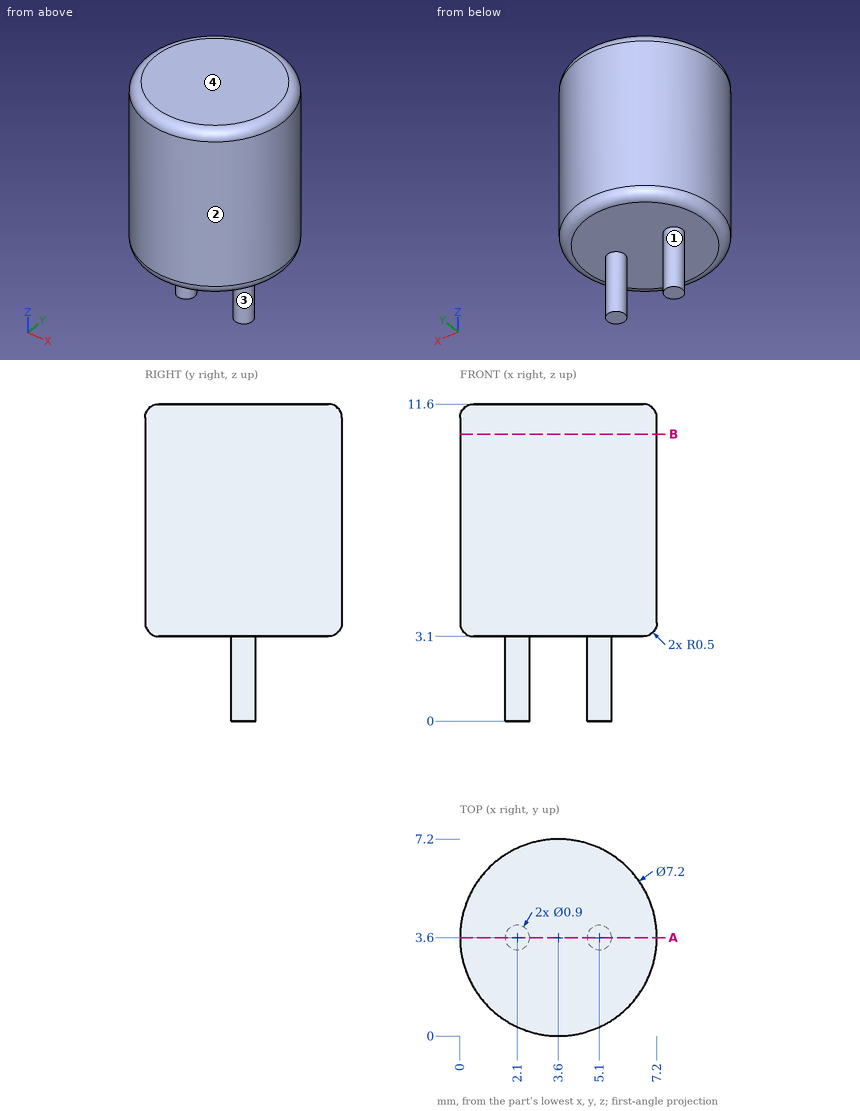
Source: three-view drawing plus pictorial views. Frame: mm from the lowest corner of the part. Give positions to 0.01 mm unless a question says otherwise; leave off trailing zeros. Order: outer loops, then holes, each group sorted by start corner. A loop starts at its lowest first (then second) coordinate and runs counter-clockwise, first axis right, second up. Notation, with made-up numbers: (45, -36) - (68, -36) arc R11 cw to (68, -32) - close; hole circle Ø2 at (48.25, 52). An arc over 180 degrees is marked (long way). Answer as a JSON object with one key per item and string values. Group by question number.
Q1. Mould query, pull axis X, two halves, no side actions, for the marked faces 1, 2, 3 and 4. Classes: pulls with the +X half, pulls with the -X half, needs draft (parallel to the pull), parting line crosses it, or undercut.
Q2. Cut plane A-A, the plane y = 3.6. Output: boundary loops of the cut face in (x, z).
Q3. First-contact query: pin 1 Ø1 at (x, y) = (2.5, 6) entering from -Z; pin 2 Ø1 at (x, z) = (1, 5) entering from +Y; pin 3 Ø1.5 at (x, z) = (5.5, 3) entering from +Y. Flat tips, straight axial feed; report the tip coordinate or a pass-through.
Q4. Cut plane B-B, the plane z = 10.5. Output: boundary loops of the cut face in (x, y), then the cut area to 3 significant figures.
Q5. Line query: probe 1 along Z at (x, y) = (2.25, 3); probe 2 along Z at (x, y) = (1.5, 6.25); probe 3 along X at (y, z) = (1.5, 6). Output: solid intervals per line, ascending.
Results:
{
 "1": {"face 1": "undercut", "face 2": "parting line crosses it", "face 3": "undercut", "face 4": "needs draft"},
 "2": {"outline": "(0, 3.6) arc R0.5 ccw to (0.5, 3.1) - (1.65, 3.1) - (1.65, 0) - (2.55, 0) - (2.55, 3.1) - (4.65, 3.1) - (4.65, 0) - (5.55, 0) - (5.55, 3.1) - (6.7, 3.1) arc R0.5 ccw to (7.2, 3.6) - (7.2, 11.1) arc R0.5 ccw to (6.7, 11.6) - (0.5, 11.6) arc R0.5 ccw to (0, 11.1) - close"},
 "3": {"pin 1": "z = 3.1", "pin 2": "y = 6.52", "pin 3": "y = 6.93"},
 "4": {"outline": "circle Ø7.2 at (3.6, 3.6)", "area": "40.7 mm^2"},
 "5": {"probe 1": "3.1 to 11.6", "probe 2": "3.19 to 11.51", "probe 3": "0.68 to 6.52"}
}
